Design review of the part shown in the three views and the two pictorial views. Dimensions are in mm from the part's minimum x, y and z. Give positions to 0.01 mm unless a question says otherwise; leave off trailing zeros. Loops run counter-clockwise (first coordinate to the right, second up) from the corner with the lowest first, then second, coordinate; pieces in that order, holes last. Notation, with made-up numbers: (54, 11.5) -> (85, 11.5) arc R30 cw to (85, 47.5) -> close; hole circle Ø8 at (61.25, 58.5). An arc over 180 degrees is marked (long way). Answer as CSV lines item,"result".
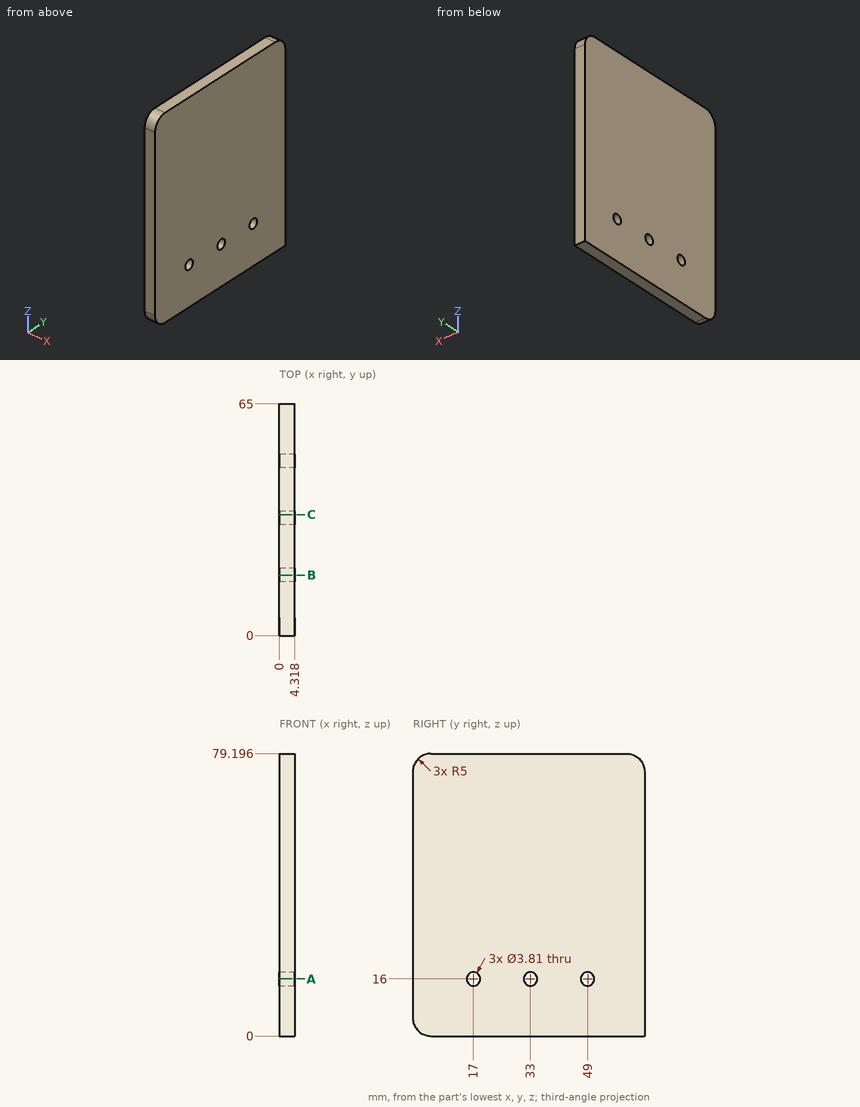
Q1. To check wall thickness, follow probe 1 along Y at (x, z) = (1.4, 16) (3 decimals); probe 2 along Z at (x, y) = (2.6, 48.5). State the ranges of each line that lie inside material, in increasing order. Write a range as from..to.
Filled sheet:
probe 1,"y = 0..15.095, 18.905..31.095, 34.905..47.095, 50.905..65"
probe 2,"z = 0..14.16, 17.84..79.2"
Q2. Clearance check with flat-ended pins moving along their axes: pin 1 Ø3.5 at (y, z) = (17, 16) entering from -X; pin 2 Ø1 at (x, z) = (4, 59.5) entering from -Y. State where each tip first meets the part, or that it passes through.
Filled sheet:
pin 1,"passes through"
pin 2,"stops at y = 0"
Q3. We need section B-B, the plane y = 17. State the section outline as (x, z) points (3 decimals).
Filled sheet:
outline,"(0, 0) -> (4.318, 0) -> (4.318, 14.095) -> (0, 14.095) -> close; (0, 17.905) -> (4.318, 17.905) -> (4.318, 79.196) -> (0, 79.196) -> close"
Q4. We need section C-C, the plane y = 34. State the section outline as (x, z) points.
Filled sheet:
outline,"(0, 0) -> (4.32, 0) -> (4.32, 14.38) -> (0, 14.38) -> close; (0, 17.62) -> (4.32, 17.62) -> (4.32, 79.2) -> (0, 79.2) -> close"
Q5. We need section A-A, the plane z = 16. State the section outline as (x, y) points (3 decimals), and give its area (3 significant figures).
Filled sheet:
outline,"(0, 0) -> (4.318, 0) -> (4.318, 15.095) -> (0, 15.095) -> close; (0, 18.905) -> (4.318, 18.905) -> (4.318, 31.095) -> (0, 31.095) -> close; (0, 34.905) -> (4.318, 34.905) -> (4.318, 47.095) -> (0, 47.095) -> close; (0, 50.905) -> (4.318, 50.905) -> (4.318, 65) -> (0, 65) -> close"
area,"231 mm^2"
